Source: three-view drawing plus pictorial views. Frame: mm from the lowest corner of the part. Give positions to 0.01 mm unless a question says otherwise; leave off trailing zeros. Loops run counter-clockwise (first coordinate to the right, second up) from the corner with the lowest first, then second, coordinate; pieces in that order, holes last. Notation, with made-up numbers: M 59.5,62.5 L 109.5,62.5 A35 ccw 109.5,101.5 Z; hole C 0,25.5 d9. An arc over 180 degrees is marked long. Put each result on its own line as item: value. Start each with the question number.
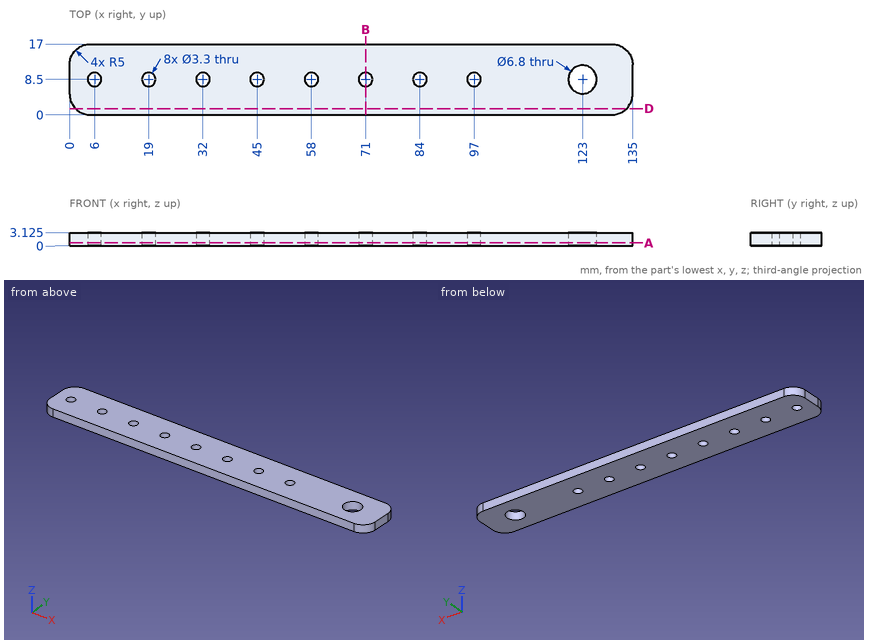
1. Contact query for a flat-ended pin moving along its axis: pin 1 (5.5 mm diameter, centred on x = 32, y = 8.5, fed in from +Z) (3 decimals). Output: stop coordinate, or through.
2. Ray query, line 1 (Y direction, x = 97, z = 1.55); line 2 (Y direction, x = 123, z = 1.95); line 3 (X direction, y = 10.5, z = 0.1). Return the intervals inside material, ascending.
3. Section D-D, the plane y = 1.5. Output: boundary loops of the cut face in (x, z) (3 decimals), plus the area to 3 significant figures.
4. Section A-A, the plane z = 0.75. State how many separate pieces and enclosed holes the cut face has, plus the area to 3 significant figures.
5. Section B-B, the plane x = 71. Output: boundary loops of the cut face in (y, z) (3 decimals).
Results found:
1. pin 1: z = 3.125
2. line 1: 0 to 6.85, 10.15 to 17
2. line 2: 0 to 5.1, 11.9 to 17
2. line 3: 0 to 120.25, 125.75 to 135
3. outline: M 1.429,0 L 133.571,0 L 133.571,3.125 L 1.429,3.125 Z
3. area: 413 mm²
4. separate pieces: 1
4. enclosed holes: 9
4. area: 2,170 mm²
5. outline: M 0,0 L 6.85,0 L 6.85,3.125 L 0,3.125 Z; M 10.15,0 L 17,0 L 17,3.125 L 10.15,3.125 Z
